from build123d import *

# Parameters (mm, degrees)
SKETCH_1_R          = 10
EXTRUDE_1_DEPTH     = 30
SKETCH_1_3_W        = 5
SKETCH_1_3_H        = 20
EXTRUDE_2_DEPTH     = 25
SKETCH_2_R          = 0.925
CUT_EXTRUDE_1_DEPTH = 38.416573868
SKETCH_3_R          = 5.05
CUT_EXTRUDE_2_DEPTH = 25


with BuildPart() as part:
    # Sketch 1 → Extrude 1 (new body)
    with BuildSketch(Plane(origin=(0, 0, 0), x_dir=(1, 0, 0), z_dir=(0, 1, 0))):
        with Locations(Location((0, 0, 0), (0, 0, 270))):
            Circle(SKETCH_1_R)
    extrude(amount=-EXTRUDE_1_DEPTH)

    # Sketch 1_3 → Extrude 2 (add)
    with BuildSketch(Plane(origin=(0, 0, 0), x_dir=(1, 0, 0), z_dir=(0, 1, 0))):
        with Locations((7.5, 0)):
            Rectangle(SKETCH_1_3_W, SKETCH_1_3_H)
    extrude(amount=EXTRUDE_2_DEPTH)

    # Sketch 2 → Cut-Extrude 1 (cut, through all)
    with BuildSketch(Plane(origin=(10, 0, 0), x_dir=(0, 0, -1), z_dir=(1, 0, 0))):
        with Locations((0, 5)):
            Circle(SKETCH_2_R)
        with Locations((3.5, 5)):
            Circle(SKETCH_2_R)
        with Locations((-3.5, 5)):
            Circle(SKETCH_2_R)
        with Locations((0, 20)):
            Circle(SKETCH_2_R)
        with Locations((-3.5, 20)):
            Circle(SKETCH_2_R)
        with Locations((3.5, 20)):
            Circle(SKETCH_2_R)
        with Locations((-7.5, 12.5)):
            Circle(SKETCH_2_R)
        with Locations((7.5, 12.5)):
            Circle(SKETCH_2_R)
        with Locations((-7.5, 9)):
            Circle(SKETCH_2_R)
        with Locations((-7.5, 16)):
            Circle(SKETCH_2_R)
        with Locations((7.5, 9)):
            Circle(SKETCH_2_R)
        with Locations((7.5, 16)):
            Circle(SKETCH_2_R)
    extrude(amount=-CUT_EXTRUDE_1_DEPTH, mode=Mode.SUBTRACT)

    # Sketch 3 → Cut-Extrude 2 (cut)
    with BuildSketch(Plane.XZ.offset(30)):
        with Locations(Location((0, 0, 0), (0, 0, 270))):
            Circle(SKETCH_3_R)
    extrude(amount=-CUT_EXTRUDE_2_DEPTH, mode=Mode.SUBTRACT)


solid = part.part
For this review, take the finished solid that the model builds, in its own axes (mm). A direction names the side the tool comes from. Give positions to 0.01 mm unless a question says otherwise; leave off trailing zeros. Loops run counter-clockwise (first coordinate to the right, second up) from the corner with the lowest first, then second, coordinate; pieces in that order, holes last. Notation, with made-up numbers: M -36,78.25 L 22,78.25 A17 ccw 22,96.25 Z; hole C 84.5,81 d4. An arc over 180 degrees is marked long. Put each result on its own line as item: value. Start each with the question number.
(1) Add section C-C, the plane z = 7.5. Write out the cut boundary in (x, y) (3 decimals), then the cut area to 3 significant figures.
(2) Machinability: for faces 1 (the flat face through (0, -5, 0)), 2 (the flat face through (8, 0, 7)), 3 (the flat face through (5, 12, 0)), which of the approach directions +Z, -Z, +X, -X, +Y, -Y give a long, thin tool a straight path to every point of the face, cutting with its end or side? Answer none if there is none.
(3) The part is to be moulded in two halves that separate along Z. For faces 4 (the flat face through (7, 12, -10)), 5 (the cylindrical face through (7.535, 4.437, -2.766)), 6 (the flat face through (2, -30, -5)), say which applies: +Z half, -Z half, draft (parallel to the pull), parting line (faces both ways), or undercut.
(4) Add section A-A, the plane y = 9. Write out the cut boundary in (x, z) (3 decimals), then the cut area to 3 significant figures.
(5) Add section B-B, the plane x = 8. Give the number of separate pieces and of enclosed holes in the cut face, then the cut area to 3 significant figures.
(6) Add section D-D, the plane y = 20. Write out the cut boundary in (x, z) (3 decimals), then the cut area to 4 significant figures.
(7) For pin 1 (2.5 mm diameter, centred on y = 20, z = 0, fed in from -X); pin 2 (1.7 mm diameter, centred on y = 5, z = 3.5, fed in from -X); pin 3 (4.5 mm diameter, centred on x = -4.5, z = -1.5, fed in from +Y); pin 4 (5 mm diameter, centred on x = -3, y = -4, fed in from -Z), all flat-tipped, find the tip position at first contact; note any pin that passes through.
(8) Wall thickness on L1, parallel to Y at x = 6.9, z = 7.5 (3 decimals); L2, parallel to X at y = 6, z = 4.75; L3, parallel to Y at x = 8.75, z = -6: over which ranges is each line inside the solid? List them lowest first.
Result:
1. outline: M -6.614,-30 L 6.614,-30 L 6.614,0 L 10,0 L 10,8.075 L 5,8.075 L 5,0 L -6.614,0 Z; M 5,9.925 L 10,9.925 L 10,11.575 L 5,11.575 Z; M 5,13.425 L 10,13.425 L 10,15.075 L 5,15.075 Z; M 5,16.925 L 10,16.925 L 10,25 L 5,25 Z
1. area: 494 mm^2
2. face 1: -Y
2. face 2: +Z, +X, -Y
2. face 3: +Z, -Z, -X, +Y
3. face 4: -Z half
3. face 5: undercut
3. face 6: draft
4. outline: M 5,-10 L 10,-10 L 10,-8.425 L 5,-8.425 Z; M 5,-6.575 L 10,-6.575 L 10,6.575 L 5,6.575 Z; M 5,8.425 L 10,8.425 L 10,10 L 5,10 Z
4. area: 81.5 mm^2
5. separate pieces: 1
5. enclosed holes: 12
5. area: 828 mm^2
6. outline: M 5,-10 L 10,-10 L 10,-4.425 L 5,-4.425 Z; M 5,-2.575 L 10,-2.575 L 10,-0.925 L 5,-0.925 Z; M 5,0.925 L 10,0.925 L 10,2.575 L 5,2.575 Z; M 5,4.425 L 10,4.425 L 10,10 L 5,10 Z
6. area: 72.25 mm^2
7. pin 1: stops at x = 5
7. pin 2: passes through
7. pin 3: stops at y = 0
7. pin 4: stops at z = -9.99
8. L1: y = 0 to 8.075, 9.925 to 11.575, 13.425 to 15.075, 16.925 to 25
8. L2: x = 5 to 10
8. L3: y = 0 to 25
